Build history of the part. All positions in model axes, mm. Face numbers are marked on the shaded views. A direction names the side the tool comes from. Round coordinates to 2 decimals unless told otherwise and drop trailing zeros. Loops run counter-clockwise (first coordinate to the right, second up) from the corner with the lowest first, then second, coordinate; pieces in that order, holes last. Notation, with made-up numbers: M 57,5 L 108,5 A17 cw 108,21 Z; hole C 29.25,41 d5. An arc over 180 degrees is marked long. Write each question's results on one line, items separated by ' | '. Start each with the question number.
```python
from build123d import *

# Parameters (mm, degrees)
SKETCH1_W               = 64
SKETCH1_H               = 23
SKETCH1_W_2             = 61
SKETCH1_H_2             = 20
BOSS_EXTRUDE1_DEPTH     = 3
SKETCH1_3_W             = 64
SKETCH1_3_H             = 23
SKETCH1_3_W_2           = 61
SKETCH1_3_H_2           = 20
BOSS_EXTRUDE2_DEPTH     = 22
FILLET1_R               = 2
FILLET2_R               = 0.5
CUT_EXTRUDE1_DEPTH      = 1.5
SKETCH3_R               = 1.1
CUT_EXTRUDE2_DEPTH      = 41.5
SKETCH4_W               = 10.5
SKETCH4_H               = 8
CUT_EXTRUDE3_DEPTH      = 46.133136386
SKETCH5_W               = 4
SKETCH5_H               = 8
CUT_EXTRUDE4_DEPTH      = 14.5
FILLET3_R               = 2
SKETCH6_R               = 3
CUT_EXTRUDE5_DEPTH      = 1.5
BOSS_EXTRUDE4_START     = -2
BOSS_EXTRUDE4_DEPTH     = 3
FILLET4_R               = 0.5
FILLET5_R               = 0.5
CUT_EXTRUDE6_DEPTH      = 47.733285782
CUT_EXTRUDE6_DEPTH_BACK = 1.5
SKETCH10_R              = 2.6


with BuildPart() as part:
    # Sketch1 → Boss-Extrude1 (new body)
    # profile 1 of 2: a face of its own
    with BuildSketch(Plane(origin=(0, 0, 0), x_dir=(1, 0, 0), z_dir=(0, 1, 0))):
        Rectangle(SKETCH1_W, SKETCH1_H)
        Rectangle(SKETCH1_W_2, SKETCH1_H_2, mode=Mode.SUBTRACT)
    # profile 2 of 2: a face of its own
    with BuildSketch(Plane(origin=(0, 0, 0), x_dir=(1, 0, 0), z_dir=(0, 1, 0))):
        Rectangle(SKETCH1_W_2, SKETCH1_H_2)
    extrude(amount=-BOSS_EXTRUDE1_DEPTH)

    # Sketch1<3> → Boss-Extrude2 (add)
    with BuildSketch(Plane(origin=(0, 0, 0), x_dir=(1, 0, 0), z_dir=(0, 1, 0))):
        Rectangle(SKETCH1_3_W, SKETCH1_3_H)
        Rectangle(SKETCH1_3_W_2, SKETCH1_3_H_2, mode=Mode.SUBTRACT)
    extrude(amount=BOSS_EXTRUDE2_DEPTH)

    # Fillet1
    fillet1_edges = [part.edges().sort_by_distance(p)[0] for p in [
        (0, -3, 11.5),
        (32, -3, 0),
        (0, -3, -11.5),
        (-32, -3, 0),
        (-32, 9.5, -11.5),
        (32, 9.5, -11.5),
        (32, 9.5, 11.5),
        (-32, 9.5, 11.5),
    ]]
    fillet(fillet1_edges, radius=FILLET1_R)

    # Fillet2
    fillet2_edges = [part.edges().sort_by_distance(p)[0] for p in [
        (-30.5, 11, 10),
        (30.5, 11, 10),
        (30.5, 11, -10),
        (-30.5, 11, -10),
    ]]
    fillet(fillet2_edges, radius=FILLET2_R)

    # Sketch2 → Cut-Extrude1 (cut)
    with BuildSketch(Plane(origin=(32, 0, 0), x_dir=(0, 0, -1), z_dir=(1, 0, 0))):
        with BuildLine():
            ThreePointArc((-2, 0), (0, 2), (2, 0))
            Line((2, 0), (-2, 0))
        make_face()
    extrude(amount=-CUT_EXTRUDE1_DEPTH, mode=Mode.SUBTRACT)

    # Sketch3 → Cut-Extrude2 (cut, through all)
    with BuildSketch(Plane(origin=(0, 0, 0), x_dir=(1, 0, 0), z_dir=(0, 1, 0))):
        with Locations(Location((19.4, 0, 0), (0, 0, 270))):
            Circle(SKETCH3_R)
        with Locations(Location((-4.6, 0, 0), (0, 0, 270))):
            Circle(SKETCH3_R)
    extrude(amount=-CUT_EXTRUDE2_DEPTH, mode=Mode.SUBTRACT)

    # Sketch4 → Cut-Extrude3 (cut, through all)
    with BuildSketch(Plane.XY.offset(11.5)):
        with Locations((-22.75, 11)):
            Rectangle(SKETCH4_W, SKETCH4_H)
    extrude(amount=-CUT_EXTRUDE3_DEPTH, mode=Mode.SUBTRACT)

    # Sketch5 → Cut-Extrude4 (cut)
    with BuildSketch(Plane.ZY.offset(32)):
        with Locations((-9.5, 11)):
            Rectangle(SKETCH5_W, SKETCH5_H)
        with Locations((9.5, 11)):
            Rectangle(SKETCH5_W, SKETCH5_H)
    extrude(amount=-CUT_EXTRUDE4_DEPTH, mode=Mode.SUBTRACT)

    # Fillet3
    fillet3_edges = [part.edges().sort_by_distance(p)[0] for p in [
        (-17.5, 7, -10.75),
        (-17.5, 15, -10.75),
        (-17.5, 7, 10.75),
        (-17.5, 15, 10.75),
        (-31.25, 7, -7.5),
        (-31.25, 15, -7.5),
        (-31.25, 15, 7.5),
        (-31.25, 7, 7.5),
    ]]
    fillet(fillet3_edges, radius=FILLET3_R)

    # Sketch6 → Cut-Extrude5 (cut)
    with BuildSketch(Plane.XZ.offset(3)):
        with Locations(Location((-4.6, 0, 0), (0, 0, 270))):
            Circle(SKETCH6_R)
        with Locations(Location((19.4, 0, 0), (0, 0, 270))):
            Circle(SKETCH6_R)
    extrude(amount=-CUT_EXTRUDE5_DEPTH, mode=Mode.SUBTRACT)

    # Sketch9 → Boss-Extrude4 (add)
    with BuildSketch(Plane.XZ.offset(3).offset(BOSS_EXTRUDE4_START)):
        with BuildLine():
            Line((-15, -11.5), (-16.5, -11.5))
            Line((-16.5, -11.5), (-16.5, -12))
            ThreePointArc((-16.5, -12), (-15.767766953, -13.767766953), (-14, -14.5))
            Line((-14, -14.5), (14, -14.5))
            ThreePointArc((14, -14.5), (15.767766953, -13.767766953), (16.5, -12))
            Line((16.5, -12), (16.5, -11.5))
            Line((16.5, -11.5), (15, -11.5))
            Line((15, -11.5), (15, -12))
            ThreePointArc((15, -12), (14.707106781, -12.707106781), (14, -13))
            Line((14, -13), (-14, -13))
            ThreePointArc((-14, -13), (-14.707106781, -12.707106781), (-15, -12))
            Line((-15, -12), (-15, -11.5))
        make_face()
    extrude(amount=-BOSS_EXTRUDE4_DEPTH)

    # Fillet4
    fillet4_edges = [part.edges().sort_by_distance(p)[0] for p in [
        (-15.767766953, -1, -13.767766953),
        (-16.5, 2, -11.75),
        (-15, -1, -11.75),
        (-14.707106781, 2, -12.707106781),
        (0, -1, -13),
        (14.707106781, -1, -12.707106781),
        (15, 2, -11.75),
        (16.5, -1, -11.75),
        (15.767766953, 2, -13.767766953),
        (0, 2, -14.5),
        (-15.767766953, 2, -13.767766953),
        (-15, 2, -11.75),
        (0, 2, -13),
        (14.707106781, 2, -12.707106781),
        (16.5, 2, -11.75),
        (0, -1, -14.5),
        (15.767766953, -1, -13.767766953),
        (15, -1, -11.75),
        (-14.707106781, -1, -12.707106781),
        (-16.5, -1, -11.75),
    ]]
    fillet(fillet4_edges, radius=FILLET4_R)

    # Fillet5
    fillet5_edges = [part.edges().sort_by_distance(p)[0] for p in [
        (16.353553391, 1.853553391, -11.5),
        (15.75, 2, -11.5),
        (15.146446609, 1.853553391, -11.5),
        (15, 0.5, -11.5),
        (15.146446609, -0.853553391, -11.5),
        (-15.75, -1, -11.5),
        (15.75, -1, -11.5),
        (16.353553391, -0.853553391, -11.5),
        (-15.146446609, 1.853553391, -11.5),
        (-15.75, 2, -11.5),
        (-16.353553391, 1.853553391, -11.5),
        (-16.5, 0.5, -11.5),
        (-16.353553391, -0.853553391, -11.5),
        (-15.146446609, -0.853553391, -11.5),
        (16.5, 0.5, -11.5),
        (-15, 0.5, -11.5),
    ]]
    fillet(fillet5_edges, radius=FILLET5_R - 0.0001)  # a hair under: the kernel refuses the full size

    # Sketch10 → Cut-Extrude6 (cut, two sides: drawn at the far end of the back side and taken through both)
    with BuildSketch(Plane.XY.offset(11.5).offset(-CUT_EXTRUDE6_DEPTH_BACK)):
        with Locations(Location((0, 9, 0), (0, 0, 180))):
            Circle(SKETCH10_R)
    extrude(amount=CUT_EXTRUDE6_DEPTH + CUT_EXTRUDE6_DEPTH_BACK, mode=Mode.SUBTRACT)


solid = part.part
```
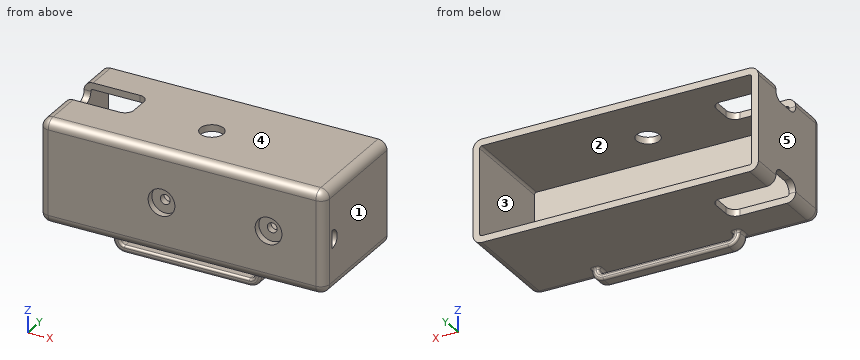
Item 1: Drop flat-ended pins along their axis: pin 1 (2 mm diameter, centred on x = 4.5, z = -13.5, fed in from +Y); pin 2 (1.5 mm diameter, centred on x = -3, z = -1, fed in from -Y); pin 3 (7 mm diameter, centred on x = 19.4, z = 0, fed in from +Y); pin 4 (10 mm diameter, centred on y = -0.5, z = -10.5, fed in from -X). Give the stop position or say it passes through.
Item 2: Mould opens along Z. For the marked faces 3, 4 and 5 say: released by +Z, released by -Z, zero draft, split by the parting line, or undercut.
Item 3: Saw through at C-C, the plane z = -3.75. Give the cut face in (x, y).
Item 4: Saw through at A-A, the plane x = 0. Give the cut face in (y, z), then the cut area to 3 significant figures.
Item 5: Saw through at D-D, the plane z = 0.5. Give the cut face in (x, y), then the cut area to 3 significant figures.
Item 6: Drill centre lines: line 1 along X through (y, z) = (-0.9, 0); line 2 along X through (y, z) = (16.5, 0.5); line 3 along X through (y, z) = (-1.9, 0). Where is each one in solid material? Low to high. Write a range as [from, to].
Item 7: Tool access for the marked faces 1 and 2: list every direction of +Z, -Z, +X, -X, +Y, -Y with a clear straight run to the whole face (end or side of a thin tool).
Item 8: Saw through at B-B, the plane y = 19. Give the cut face in (x, z), then the cut area to 3 significant figures.
Working result:
1) pin 1: stops at y = 2 | pin 2: stops at y = -1.5 | pin 3: stops at y = 0 | pin 4: stops at x = -32
2) face 3: undercut | face 4: released by +Z | face 5: zero draft
3) outline: M -32,-1 A2 ccw -30,-3 L 30,-3 A2 ccw 32,-1 L 32,22 L 30.5,22 L 30.5,0 L -30.5,0 L -30.5,22 L -32,22 Z
4) outline: M -3,-9.5 A2 ccw -1,-11.5 L 22,-11.5 L 22,-10 L 0,-10 L 0,10 L 6.4,10 L 6.4,11.5 L -1,11.5 A2 ccw -3,9.5 Z; M -1,-14 A0.5 ccw -0.5,-14.5 L 1.5,-14.5 A0.5 ccw 2,-14 L 2,-13.5 A0.5 ccw 1.5,-13 L -0.5,-13 A0.5 ccw -1,-13.5 Z; M 11.6,10 L 22,10 L 22,11.5 L 11.6,11.5 Z | area: 130 mm²
5) outline: M -32,-1 A2 ccw -30,-3 L -7.56,-3 L -7.56,-1.5 L -5.58,-1.5 L -5.58,0 L -30.5,0 L -30.5,22 L -32,22 Z; M -3.62,-1.5 L -1.64,-1.5 L -1.64,-3 L 16.44,-3 L 16.44,-1.5 L 18.42,-1.5 L 18.42,0 L -3.62,0 Z; M 20.38,-1.5 L 22.36,-1.5 L 22.36,-3 L 30,-3 A2 ccw 32,-1 L 32,0 L 20.38,0 Z; M 30.5,1.94 L 32,1.94 L 32,22 L 30.5,22 Z | area: 230 mm²
6) line 1: x = [-32, -5.7], [-3.5, 18.3], [20.5, 32] | line 2: x = [-32, -30.5], [30.5, 32] | line 3: x = [-31.79, -7.6], [-1.6, 16.4], [22.4, 31.79]
7) face 1: +Z, -Z, +X, +Y, -Y | face 2: +Y
8) outline: M -32,-9.5 A2 ccw -30,-11.5 L 30,-11.5 A2 ccw 32,-9.5 L 32,9.5 A2 ccw 30,11.5 L -30,11.5 A2 ccw -32,9.5 Z; hole M -30.5,-9.5 A0.5 ccw -30,-10 L 30,-10 A0.5 ccw 30.5,-9.5 L 30.5,9.5 A0.5 ccw 30,10 L -30,10 A0.5 ccw -30.5,9.5 Z | area: 249 mm²
